```python
from build123d import *

# Parameters (mm, degrees)
SKETCH1_R                = 50.8
BOSS_EXTRUDE1_DEPTH      = 1030
BOSS_EXTRUDE1_DEPTH_BACK = 680
SKETCH2_R                = 570
BOSS_EXTRUDE2_DEPTH      = 20
BOSS_EXTRUDE3_START      = -280
SKETCH7_R                = 305
BOSS_EXTRUDE3_DEPTH      = 620
SKETCH8_R                = 225
BOSS_EXTRUDE4_DEPTH      = 50


with BuildPart() as part:
    # Sketch1 → Boss-Extrude1 (new body, two sides)
    with BuildSketch(Plane.XY) as boss_extrude1_sk:
        Circle(SKETCH1_R)
    extrude(amount=BOSS_EXTRUDE1_DEPTH)
    extrude(boss_extrude1_sk.sketch, amount=-BOSS_EXTRUDE1_DEPTH_BACK)

    # Sketch2 → Boss-Extrude2 (add)
    with BuildSketch(Plane.XY.offset(-680)):
        Circle(SKETCH2_R)
    extrude(amount=BOSS_EXTRUDE2_DEPTH)

    # Sketch7 → Boss-Extrude3 (add)
    with BuildSketch(Plane.XY.offset(1030).offset(BOSS_EXTRUDE3_START)):
        Circle(SKETCH7_R)
    extrude(amount=-BOSS_EXTRUDE3_DEPTH)

    # Sketch8 → Boss-Extrude4 (add)
    with BuildSketch(Plane(origin=(0, 0, 130), x_dir=(-1, 0, 0), z_dir=(0, 0, -1))):
        Circle(SKETCH8_R)
    extrude(amount=BOSS_EXTRUDE4_DEPTH)


solid = part.part
```
Geometry check sheet. Reference: the model listing, model coordinates, mm. A direction names the side the tool comes from. Give positions to 0.01 mm unless a question says otherwise; leave off trailing zeros. Order: outer loops, then holes, each group sorted by start corner. A loop starts at its lowest first (then second) coordinate and runs counter-clockwise, first axis right, second up. Notation, with made-up numbers: (21.25, 67) - (41.25, 67) arc R29 cw to (41.25, 89) - close; hole circle Ø5 at (29.5, 75.25). An arc over 180 degrees is marked (long way). Answer in a Markdown table with one row per item. Add a question column.
Q1. Cross-section at D-D, the plane y = -360. Enter the section's corners in (x, z).
Q2. Gauge pin test, flat ends, axial feed: pin 1 (6 mm diameter, centred on y = -266, z = 630.5, fed in from -X); pin 2 (1.5 mm diameter, centred on x = 210.5, z = 609, fed in from +Y); pin 3 (12 mm diameter, centred on x = 69, y = 382.5, fed in from +Z). Record the tip position at first contact, or that the pin passes through.
Q3. Tool access check on faces 4 (the cylindrical face through (-11.012, -49.592, 891.96)), 5 (the flat face through (-24, -225, 130)), 6 (the flat face through (-1, 1, 1030)). Record the directions out of +Z, -Z, +X, -X, +Y, -Y that give a thin tool (end or side, any length) a straight path to the whole face; none if there is none.
Q4. Mould release check, pull along Z, two halves, no side actions. Record for faces 1 (the flat face through (53, 3, 80)), 2 (the cylindrical face through (-304.705, 13.41, 444.34)), 3 (the flat face through (-8, 8, -680)): pulls with the +Z half, pulls with the -Z half, needs draft (parallel to the pull), parting line crosses it, or undercut.
Q5. Cross-section at B-B, the plane y = 104. Enter the section's corners in (x, z), then the cut area to 3 significant figures.
Q6. Material ranges on probe 1 along Z at (x, y) = (3.5, -245.5); probe 2 along Z at (x, y) = (86, 181); probe 3 along Z at (x, y) = (-66, -406), recorded low to high. Write a range as from..to.
Q7. Cross-section at C-C, the plane z = 808. Enter the section's corners in (x, y).
Q8. Cross-section at A-A, the plane x = 103. Enter the section's corners in (y, z), then the cut area to 3 significant figures.
Check values:
| question | item | result |
|---|---|---|
| 1 | outline | (-441.93, -680) - (441.93, -680) - (441.93, -660) - (-441.93, -660) - close |
| 2 | pin 1 | stops at x = -154.45 |
| 2 | pin 2 | stops at y = 221.43 |
| 2 | pin 3 | stops at z = -660 |
| 3 | face 4 | +Z |
| 3 | face 5 | none |
| 3 | face 6 | +Z, +X, -X, +Y, -Y |
| 4 | face 1 | undercut |
| 4 | face 2 | needs draft |
| 4 | face 3 | pulls with the -Z half |
| 5 | outline | (-560.43, -680) - (560.43, -680) - (560.43, -660) - (-560.43, -660) - close; (-286.72, 130) - (-199.52, 130) - (-199.52, 80) - (199.52, 80) - (199.52, 130) - (286.72, 130) - (286.72, 750) - (-286.72, 750) - close |
| 5 | area | 398,000 mm^2 |
| 6 | probe 1 | z = -680..-660, 130..750 |
| 6 | probe 2 | z = -680..-660, 80..750 |
| 6 | probe 3 | z = -680..-660 |
| 7 | outline | circle Ø101.6 at (0, 0) |
| 8 | outline | (-560.62, -680) - (560.62, -680) - (560.62, -660) - (-560.62, -660) - close; (-287.08, 130) - (-200.04, 130) - (-200.04, 80) - (200.04, 80) - (200.04, 130) - (287.08, 130) - (287.08, 750) - (-287.08, 750) - close |
| 8 | area | 398,000 mm^2 |
